Autodesk Inventor part; units mm, degrees
ref_plane "YZ Plane" through (0, 0, 0) normal (1, 0, 0) x (0, 1, 0)
ref_plane "XZ Plane" through (0, 0, 0) normal (0, 1, 0) x (-1, 0, 0)
ref_plane "XY Plane" through (0, 0, 0) normal (0, 0, 1) x (1, 0, 0)
ref_plane "Work Plane1" through (0, 0, 0) normal (0, 0, 1) x (1, 0, 0)
sketch "Sketch1" plane through (0, 0, 0) normal (0, 0, 1) x (1, 0, 0)
  line L0 (13.075, 9.425) -> (13.075, -9.425)
  arc A0 (13.075, 9.425) -> (9.075, 13.425) centre (9.075, 9.425) ccw
  line L1 (5, 13.425) -> (9.075, 13.425)
  line L2 (-4, 13.425) -> (4, 13.425)
  line L3 (5, 13.425) -> (4, 13.425)
  line L4 (-4, 13.425) -> (-5, 13.425)
  line L5 (-9.075, 13.425) -> (-5, 13.425)
  arc A1 (-9.075, 13.425) -> (-13.075, 9.425) centre (-9.075, 9.425) ccw
  line L6 (-13.075, -9.425) -> (-13.075, 9.425)
  arc A2 (-13.075, -9.425) -> (-9.075, -13.425) centre (-9.075, -9.425) ccw
  line L7 (9.075, -13.425) -> (-9.075, -13.425)
  arc A3 (9.075, -13.425) -> (13.075, -9.425) centre (9.075, -9.425) ccw
  point P0 (0, 0)
extrude "Extrusion1" add sketch "Sketch1" along normal blind 1.2
sketch "Sketch2" plane through (0, 0, 1.2) normal (0, 0, 1) x (1, 0, 0)
  circle A0 centre (0, -2) radius 3.85
  line L0 (-9.075, -13.425) -> (9.075, -13.425)
  point P0 (0, 0)
  dimension "d10" = 13.425
  dimension "d11" = 2
extrude "Extrusion2" cut sketch "Sketch2" against normal blind 1.2
sketch "Sketch3" plane through (0, 0, 0) normal (0, 0, -1) x (-1, 0, 0)
  arc A0 (-9.075, 12.225) -> (-11.875, 9.425) centre (-9.075, 9.425) ccw
  line L0 (-9.075, 12.225) -> (-5, 12.225)
  line L1 (-11.875, -9.425) -> (-11.875, 9.425)
  arc A1 (-11.875, -9.425) -> (-9.075, -12.225) centre (-9.075, -9.425) ccw
  line L2 (9.075, -12.225) -> (-9.075, -12.225)
  arc A2 (9.075, -12.225) -> (11.875, -9.425) centre (9.075, -9.425) ccw
  line L3 (11.875, 9.425) -> (11.875, -9.425)
  arc A3 (11.875, 9.425) -> (9.075, 12.225) centre (9.075, 9.425) ccw
  line L4 (5, 12.225) -> (9.075, 12.225)
  line L5 (5, 12.125) -> (9.075, 12.125)
  arc A4 (11.775, 9.425) -> (9.075, 12.125) centre (9.075, 9.425) ccw
  line L6 (11.775, 9.425) -> (11.775, -9.425)
  arc A5 (9.075, -12.125) -> (11.775, -9.425) centre (9.075, -9.425) ccw
  line L7 (9.075, -12.125) -> (-9.075, -12.125)
  arc A6 (-11.775, -9.425) -> (-9.075, -12.125) centre (-9.075, -9.425) ccw
  line L8 (-11.775, -9.425) -> (-11.775, 9.425)
  arc A7 (-9.075, 12.125) -> (-11.775, 9.425) centre (-9.075, 9.425) ccw
  line L9 (-9.075, 12.125) -> (-5, 12.125)
  line L10 (5, 11.125) -> (9.075, 11.125)
  arc A8 (10.775, 9.425) -> (9.075, 11.125) centre (9.075, 9.425) ccw
  line L11 (10.775, 9.425) -> (10.775, -9.425)
  arc A9 (9.075, -11.125) -> (10.775, -9.425) centre (9.075, -9.425) ccw
  line L12 (9.075, -11.125) -> (-9.075, -11.125)
  arc A10 (-10.775, -9.425) -> (-9.075, -11.125) centre (-9.075, -9.425) ccw
  line L13 (-10.775, -9.425) -> (-10.775, 9.425)
  arc A11 (-9.075, 11.125) -> (-10.775, 9.425) centre (-9.075, 9.425) ccw
  line L14 (-9.075, 11.125) -> (-5, 11.125)
  line L15 (-5, 12.125) -> (-5, 11.125)
  line L16 (5, 12.125) -> (5, 11.125)
  point P0 (0, 0)
  dimension "d5" = 0.1
  dimension "d6" = 1
extrude "Extrusion3" add sketch "Sketch3" along normal blind 5
sketch "Sketch4" plane through (0, 0, 1.2) normal (0, 0, 1) x (1, 0, 0)
  circle A0 centre (0, -2) radius 3.85 construction
  circle A1 centre (0, -2) radius 5
  point P0 (0, 0)
  dimension "d12" = 10
extrude "Extrusion4" cut sketch "Sketch4" against normal blind 10
sketch "Sketch5" plane through (0, 0, 1.2) normal (0, 0, 1) x (1, 0, 0)
  circle A0 centre (0, -2) radius 5
  line L0 (13.075, -9.425) -> (13.075, 9.425)
  arc A1 (13.075, 9.425) -> (9.075, 13.425) centre (9.075, 9.425) ccw
  line L1 (9.075, 13.425) -> (-9.075, 13.425)
  arc A2 (-9.075, 13.425) -> (-13.075, 9.425) centre (-9.075, 9.425) ccw
  line L2 (-13.075, 9.425) -> (-13.075, -9.425)
  arc A3 (-13.075, -9.425) -> (-9.075, -13.425) centre (-9.075, -9.425) ccw
  line L3 (-9.075, -13.425) -> (9.075, -13.425)
  arc A4 (9.075, -13.425) -> (13.075, -9.425) centre (9.075, -9.425) ccw
  point P0 (0, 0)
extrude "Extrusion5" add sketch "Sketch5" along normal blind 1
sketch "Sketch6" plane through (0, 0, 0) normal (0, 0, -1) x (-1, 0, 0)
  arc A0 (-9.075, 13.425) -> (-13.075, 9.425) centre (-9.075, 9.425) ccw
  line L0 (-13.075, 9.425) -> (-13.075, -9.425)
  arc A1 (-13.075, -9.425) -> (-9.075, -13.425) centre (-9.075, -9.425) ccw
  line L1 (-9.075, -13.425) -> (9.075, -13.425)
  arc A2 (9.075, -13.425) -> (13.075, -9.425) centre (9.075, -9.425) ccw
  line L2 (13.075, -9.425) -> (13.075, 9.425)
  arc A3 (13.075, 9.425) -> (9.075, 13.425) centre (9.075, 9.425) ccw
  line L3 (9.075, 13.425) -> (-9.075, 13.425)
  line L4 (-5, 12.125) -> (-9.075, 12.125)
  arc A4 (-9.075, 12.125) -> (-11.775, 9.425) centre (-9.075, 9.425) ccw
  line L5 (-11.775, 9.425) -> (-11.775, -9.425)
  arc A5 (-11.775, -9.425) -> (-9.075, -12.125) centre (-9.075, -9.425) ccw
  line L6 (-9.075, -12.125) -> (9.075, -12.125)
  arc A6 (9.075, -12.125) -> (11.775, -9.425) centre (9.075, -9.425) ccw
  line L7 (11.775, -9.425) -> (11.775, 9.425)
  arc A7 (11.775, 9.425) -> (9.075, 12.125) centre (9.075, 9.425) ccw
  line L8 (9.075, 12.125) -> (5, 12.125)
  line L9 (-5, 12.125) -> (5, 12.125)
  point P0 (0, 0)
extrude "Extrusion6" add sketch "Sketch6" along normal blind 0.8
sketch "Sketch7" plane through (0, 0, 2.2) normal (0, 0, 1) x (1, 0, 0)
  line L0 (-4.3978, 12.3352) -> (4.3978, 12.3352) construction
  line L1 (4.3978, 12.3352) -> (4.3978, 5.3989) construction
  line L2 (4.3978, 5.3989) -> (-4.3978, 5.3989) construction
  line L3 (-4.3978, 5.3989) -> (-4.3978, 12.3352) construction
  line L4 (0, -18.795) -> (0, 18.795)
  spline S0 degree 2 poles (-2.3788, 10.9588) (-1.9786, 11.3515) (-1.3128, 11.4189) (-1.2418, 11.086) knots 0 0 0 1 2 2 2
  spline S1 degree 2 poles (-1.2418, 11.086) (-1.1857, 10.798) (-1.657, 10.3753) knots 0 0 0 1 1 1
  spline S2 degree 2 poles (-1.657, 10.3753) (-2.3452, 9.7432) (-2.6444, 8.1947) (-2.2292, 7.4055) knots 0 0 0 1 2 2 2
  spline S3 degree 2 poles (-2.2292, 7.4055) (-1.93, 6.8557) (-0.6807, 6.0627) (0.475, 6.0627) (1.728, 6.8557) (2.0123, 7.4055) knots 0 0 0 1 2 3 4 4 4
  spline S4 degree 2 poles (2.0123, 7.4055) (2.4387, 8.1947) (2.1507, 9.732) (1.4625, 10.3641) knots 0 0 0 1 2 2 2
  spline S5 degree 2 poles (1.4625, 10.3641) (1.0735, 10.7194) (1.0286, 11.3403) (1.4064, 11.3964) knots 0 0 0 1 2 2 2
  spline S6 degree 2 poles (1.4064, 11.3964) (1.657, 11.4301) (2.6444, 10.5474) (2.895, 10.0424) knots 0 0 0 1 2 2 2
  spline S7 degree 2 poles (2.895, 10.0424) (3.355, 9.1597) (3.0222, 6.9342) (2.3115, 6.2124) knots 0 0 0 1 2 2 2
  spline S8 degree 2 poles (2.3115, 6.2124) (1.7841, 5.6625) (0.4301, 5.1464) (-0.8752, 5.2137) (-2.1133, 5.7785) (-3.0109, 6.7061) (-3.4897, 8.0488) (-3.4112, 8.8044) knots 0 0 0 1 2 3 4 5 6 6 6
  spline S9 degree 2 poles (-3.4112, 8.8044) (-3.3289, 9.515) (-2.8838, 10.4688) (-2.3788, 10.9588) knots 0 0 0 1 2 2 2
  spline S10 degree 2 poles (-0.7518, 10.1584) (-0.7855, 11.935) (-0.6246, 12.3352) (-0.0636, 12.2903) knots 0 0 0 1 2 2 2
  line L5 (-0.0636, 12.2903) -> (0.49, 12.2455)
  line L6 (0.49, 12.2455) -> (0.49, 10.308)
  line L7 (0.49, 10.308) -> (0.49, 8.3668)
  line L8 (0.49, 8.3668) -> (-0.1085, 8.3668)
  line L9 (-0.1085, 8.3668) -> (-0.7032, 8.3668)
  line L10 (-0.7032, 8.3668) -> (-0.7518, 10.1584)
  point P0 (0, 0)
  point P1 (0, 12.3352)
extrude "Extrusion7" cut sketch "Sketch7" against normal blind 1
properties part number "cap"
CAD build for the part. Positions are in the model's coordinates, mm. A direction names the side the tool comes from. Coordinates: 2 decimals unless noted, no trailing zeros. Order: outer loops, then holes, each group sorted by start corner. A loop starts at its lowest first (then second) coordinate and runs counter-clockwise, first axis right, second up. Notation, with made-up numbers: (22, 28.5) -> (44, 28.5) arc R28 ccw to (44, 51.5) -> close; hole circle Ø7 at (-16, 17). An arc over 180 degrees is marked (long way). Answer in a Markdown table with one row per item.
1) Band-saw the part on A-A (y = -2). List the corners of the cut face in (x, z) (3 decimals), and give its area (3 significant figures).
Check values:
| item | result |
|---|---|
| outline | (-13.075, -0.8) -> (-11.775, -0.8) -> (-11.775, -5) -> (-10.775, -5) -> (-10.775, 0) -> (-5, 0) -> (-5, 2.2) -> (-13.075, 2.2) -> close; (5, 0) -> (10.775, 0) -> (10.775, -5) -> (11.775, -5) -> (11.775, -0.8) -> (13.075, -0.8) -> (13.075, 2.2) -> (5, 2.2) -> close |
| area | 47.6 mm2 |
2) Mould opens along Y. For faces 1 (the face through (11.934, 12.222, 0.721)), 2 (the face through (1, -13, -0.8)), 3 (the face through (-11.934, -12.222, 0.721)), 4 (the face through (-10.775, 0, -2)) say: pulls with the +Y half, pulls with the -Y half, needs draft (parallel to the pull), parting line crosses it, or undercut.
Check values:
| item | result |
|---|---|
| face 1 | pulls with the +Y half |
| face 2 | needs draft |
| face 3 | pulls with the -Y half |
| face 4 | undercut |
3) Band-saw the part on C-C (y = 3.5). List the corners of the cut face in (x, z) (3 decimals), and give its area (3 significant figures).
Check values:
| item | result |
|---|---|
| outline | (-13.075, -0.8) -> (-11.775, -0.8) -> (-11.775, -5) -> (-10.775, -5) -> (-10.775, 0) -> (10.775, 0) -> (10.775, -5) -> (11.775, -5) -> (11.775, -0.8) -> (13.075, -0.8) -> (13.075, 2.2) -> (-13.075, 2.2) -> close |
| area | 69.6 mm2 |
4) Band-saw the part on B-B (x = 5.75). List the corners of the cut face in (y, z) (3 decimals).
Check values:
| item | result |
|---|---|
| outline | (-13.425, -0.8) -> (-12.125, -0.8) -> (-12.125, -5) -> (-11.125, -5) -> (-11.125, 0) -> (11.125, 0) -> (11.125, -5) -> (12.125, -5) -> (12.125, -0.8) -> (13.425, -0.8) -> (13.425, 2.2) -> (-13.425, 2.2) -> close |
5) Which spindle directions (+Z, -Z, +X, -X, +Y, -Y) get a long thin tool onto all of the face, cutting with end or side? Do faces 5 (the face through (-13.075, 0, 1)), 6 (the face through (0, -12.125, -3)), 7 (the face through (10.264, -10.64, -2.465)), 8 (the face through (-11.01, -11.31, -2.87)), 9 (the face through (-7, 12.125, -3)). Say none if no direction does.
Check values:
| item | result |
|---|---|
| face 5 | +Z, -Z, -X, +Y, -Y |
| face 6 | -Z, +X, -X, -Y |
| face 7 | -Z |
| face 8 | -Z, -X, -Y |
| face 9 | -Z, +X, -X, +Y |
6) Drill centre lines: line 1 (Y direction, x = 0, z = 1.7) (3 decimals); line 2 (Y direction, x = 0, z = 0.8) (3 decimals); line 3 (Y direction, x = 6.75, z = -3) (3 decimals). Where is each one in solid material? Low to high.
Check values:
| item | result |
|---|---|
| line 1 | -13.425 to -7, 3 to 5.177, 6.066 to 8.367, 12.285 to 13.425 |
| line 2 | -13.425 to -7, 3 to 13.425 |
| line 3 | -12.125 to -11.125, 11.125 to 12.125 |
7) Flat gauge pins, fed straight in: P1, Ø3, axis at y = 10, z = 0.5, coming from the -X side (3 decimals); P2, Ø2, axis at x = -3.5, z = -2.5, coming from the -Y side (3 decimals); P3, Ø1.1, axis at y = 11.5, z = 1.5, coming from the -X side; P4, Ø4, axis at x = 8, z = -3, coming from the +Y side (3 decimals). Where does each tip first touch, or does it go through?
Check values:
| item | result |
|---|---|
| P1 | x = -13.075 |
| P2 | y = -12.125 |
| P3 | x = -12.77 |
| P4 | y = 12.125 |
